Could you check a few things on this model? Use its own coordinates, in mm. A direction names the side the tool comes from. Give positions to 0.01 mm unless a question says otherwise; leave off trailing zeros. Return JSON: item names as keys, results as strings. Group by question number.
1. If we mould it in two halves opening along X, with no side actions, what happens to faces 1 (the cylindrical face through (-1.5, 0.07, 3.52)), 2 (the cylindrical face through (0.54, -2.44, 0.99)), 3 (the flat face through (-2, 0, 5))? For each: +X half, -X half, draft (parallel to the pull), parting line (faces both ways), or undercut.
2. For faces 4 (the flat face through (0, -2, 2)), 5 (the flat face through (-3, -2, 0)), which set-ups out of +Z, -Z, +X, -X, +Y, -Y let a thin tool reach every point of the face, with its end or its side?
3. For pin 1 (3 mm diameter, centred on x = -2, z = 3, fed in from +Y); pin 2 (2 mm diameter, centred on y = -5, z = 3.5, fed in from -X); pin 3 (1.5 mm diameter, centred on x = 0.5, z = 0.5, fed in from +Y), each with a flat end and sliding along its axis, tell me the tip position at first contact or that it passes through.
4. Please list where these lines run through material, in increasing order: line 1 (Y direction, x = -1, z = 2.45) (3 decimals); line 2 (Y direction, x = 0, z = 2.75) (3 decimals); line 3 (Z direction, x = 4.25, y = 0.5).
```python
from build123d import *

# Parameters (mm, degrees)
CROQUIS10_R           = 1.5
CORTAR_EXTRUIR1_DEPTH = 5
CROQUIS11_R           = 2.5
CORTAR_EXTRUIR2_DEPTH = 2


with BuildPart() as part:
    # Croquis1 → Recubrir1 section 0
    with BuildSketch(Plane.XY):
        with BuildLine():
            Line((-5, -10), (5, -10))
            Line((5, -10), (5, 10))
            Line((5, 10), (-5, 10))
            Line((-5, 10), (-5, -10))
        make_face()
    # Croquis9 → Recubrir1 section 1
    with BuildSketch(Plane.XY.offset(5)):
        with BuildLine():
            Line((-2.5, 2.5), (2.5, 2.5))
            Line((2.5, 2.5), (2.5, -2.5))
            Line((2.5, -2.5), (-2.5, -2.5))
            Line((-2.5, -2.5), (-2.5, 2.5))
        make_face()
    loft()

    # Croquis10 → Cortar-Extruir1 (cut)
    with BuildSketch(Plane.XY.offset(5)):
        Circle(CROQUIS10_R)
    extrude(amount=-CORTAR_EXTRUIR1_DEPTH, mode=Mode.SUBTRACT)

    # Croquis11 → Cortar-Extruir2 (cut)
    with BuildSketch(Plane(origin=(0, 0, 0), x_dir=(-1, 0, 0), z_dir=(0, 0, -1))):
        Circle(CROQUIS11_R)
    extrude(amount=-CORTAR_EXTRUIR2_DEPTH, mode=Mode.SUBTRACT)


solid = part.part
```
Answer:
{
 "1": {"face 1": "undercut", "face 2": "undercut", "face 3": "draft"},
 "2": {"face 4": "-Z", "face 5": "-Z, +X, -X, +Y, -Y"},
 "3": {"pin 1": "stops at y = 7.75", "pin 2": "stops at x = -3.75", "pin 3": "stops at y = 10"},
 "4": {"line 1": "y = -6.325 to -1.118, 1.118 to 6.325", "line 2": "y = -5.875 to -1.5, 1.5 to 5.875", "line 3": "z = 0 to 1.5"}
}
